Answer from the drawing. Dimensions are ordinates in mm from the lowest x, y and z of the part. A direction names the side the tool comes from. Coordinates: 2 decimals unless noted, no trailing zeros. Write each loop counter-clockwise with the first axis right and the second up, starting at its lowest first coordinate (ties: lowest second). Pieces come first, ordered by that corner, then holes.
(1) Straight lines are drawn through the part: line 1 (Y direction, x = 39.5, z = 3) (1 decimal); line 2 (X direction, y = 24, z = 11.75); line 3 (X direction, y = 17.5, z = 7). For each, find the intervals that lie inside material, in ascending order.
(2) The part is cut by section B-B on x = 47. Determine the outline of the cut face in (y, z), plus the area to 3 significant figures.
(3) For a pull along Y with two mould halves and no side action, classify the marked faces 3, 4 and 5 as +Y half, -Y half, draft (parallel to the pull), parting line (faces both ways), or undercut.
(4) The part is cut by section A-A on z = 5. Give the number of separate pieces and of enclosed holes in the cut face, plus the area to 3 significant figures.
(5) Given P1, Ø1, axis at x = 37.5, z = 3, coming from the +Y side; P2, Ø6, axis at y = 36.5, z = 3.5, coming from the +X side; P3, Ø5, axis at x = 27.5, y = 39.5, coming from the +Z side, each flat-ended and moving along its own axis, determine where each tip first touches the part or whether it passes through.
(6) Which of the six approach directions +Z, -Z, +X, -X, +Y, -Y give full straight-line access (tool end or side, diameter ignored) to the marked faces 1 and 2?
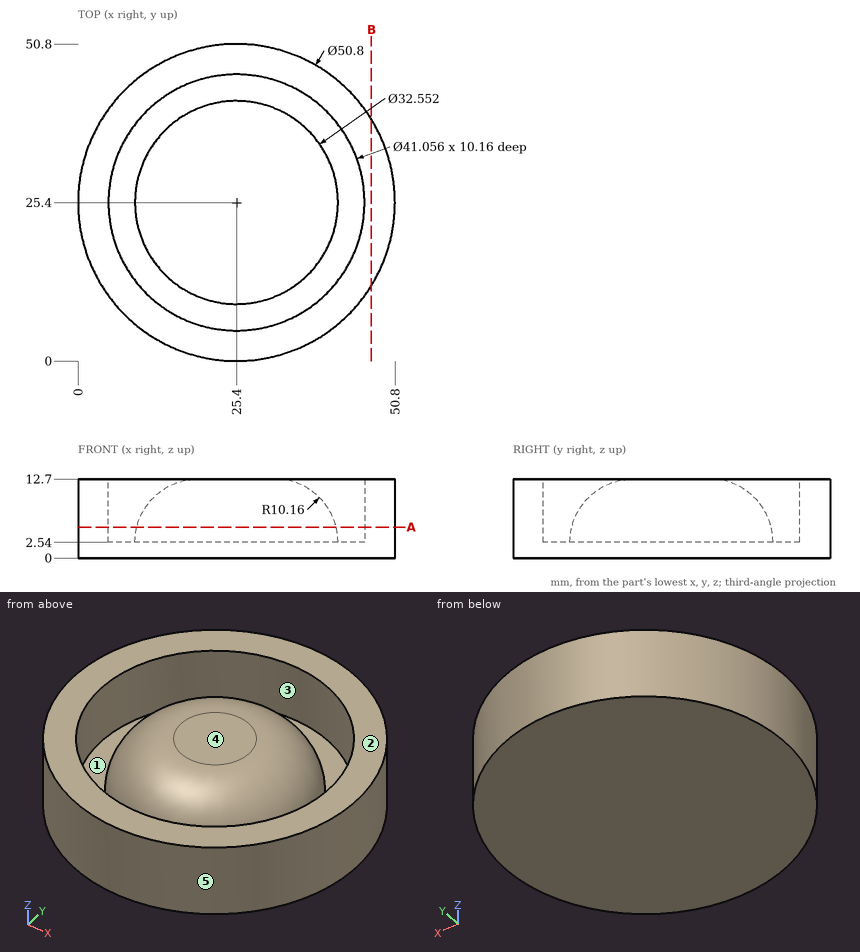
Model answer:
1. line 1: y = 4.3 to 10.5, 17.3 to 33.5, 40.3 to 46.5
1. line 2: x = 0.04 to 4.92, 15.09 to 35.71, 45.88 to 50.76
1. line 3: x = 1.26 to 6.45, 12.36 to 38.44, 44.35 to 49.54
2. outline: (12.04, 0) - (38.76, 0) - (38.76, 12.7) - (12.04, 12.7) - close
2. area: 339 mm2
3. face 3: undercut
3. face 4: draft
3. face 5: parting line
4. separate pieces: 2
4. enclosed holes: 1
4. area: 1,500 mm2
5. P1: stops at y = 48
5. P2: stops at x = 49.47
5. P3: stops at z = 10.99
6. face 1: +Z
6. face 2: +Z, +X, -X, +Y, -Y
